```python
from build123d import *

# Parameters (mm, degrees)
F1_DEPTH       = 7
F3_DEPTH       = 5
F5_D           = 5.5
F5_CSINK_D     = 11.2
F5_CSINK_ANGLE = 90
F6_R           = 8
F7_R           = 3
F8_SIZE        = 1


with BuildPart() as f1:
    # F0 (on Top) → F1 (new body)
    with BuildSketch(Plane.XY):
        with BuildLine():
            Line((12.409673646, 7.5), (-12.409673646, 7.5))
            ThreePointArc((-12.409673646, 7.5), (-14.5, 0), (-12.409673646, -7.5))
            Line((-12.409673646, -7.5), (12.409673646, -7.5))
            ThreePointArc((12.409673646, -7.5), (14.5, 0), (12.409673646, 7.5))
        make_face()
    extrude(amount=F1_DEPTH)

    # F2 (on face) → F3 (join)
    with BuildSketch(Plane(origin=(0, 0, 0), x_dir=(1, 0, 0), z_dir=(0, 0, -1))):
        with BuildLine():
            Line((14.9666296342, 12.5000001863), (-14.9666296342, 12.5000001863))
            ThreePointArc((-14.9666296342, 12.5000001863), (-19.5000001863, 0), (-14.9666296342, -12.5000001863))
            Line((-14.9666296342, -12.5000001863), (14.9666296342, -12.5000001863))
            ThreePointArc((14.9666296342, -12.5000001863), (19.5000001863, 0), (14.9666296342, 12.5000001863))
        make_face()
        with BuildLine():
            Line((-12.409673646, 7.5), (12.409673646, 7.5))
            ThreePointArc((12.409673646, 7.5), (14.5, 0), (12.409673646, -7.5))
            Line((12.409673646, -7.5), (-12.409673646, -7.5))
            ThreePointArc((-12.409673646, -7.5), (-14.5, 0), (-12.409673646, 7.5))
        make_face(mode=Mode.SUBTRACT)
        with BuildLine():
            ThreePointArc((12.409673646, -7.5), (14.5, 0), (12.409673646, 7.5))
            Line((12.409673646, 7.5), (-12.409673646, 7.5))
            ThreePointArc((-12.409673646, 7.5), (-14.5, 0), (-12.409673646, -7.5))
            Line((-12.409673646, -7.5), (12.409673646, -7.5))
        make_face()
    extrude(amount=F3_DEPTH)

    # F5 (through all)
    with Locations(Plane(origin=(0, 0, -5), x_dir=(1, 0, 0), z_dir=(0, 0, -1))):
        with Locations((-8, 0), (8, 0)):
            CounterSinkHole(F5_D / 2, F5_CSINK_D / 2, counter_sink_angle=F5_CSINK_ANGLE)

    # F6
    f6_edges = [f1.edges().sort_by_distance(p)[0] for p in [
        (14.96663, -12.5, -2.5),
        (14.96663, 12.5, -2.5),
        (-14.96663, 12.5, -2.5),
        (-14.96663, -12.5, -2.5),
    ]]
    fillet(f6_edges, radius=F6_R)

    # F7
    f7_edges = [f1.edges().sort_by_distance(p)[0] for p in [
        (12.409674, -7.5, 3.5),
        (12.409674, 7.5, 3.5),
        (-12.409674, 7.5, 3.5),
        (-12.409674, -7.5, 3.5),
    ]]
    fillet(f7_edges, radius=F7_R)

    # F8
    f8_edges = [f1.edges().sort_by_distance(p)[0] for p in [
        (0, -12.5, -5),
        (-19.5, 0, -5),
        (0, 12.5, -5),
        (19.5, 0, -5),
        (19.5, 0, 0),
        (0, -12.5, 0),
        (-19.5, 0, 0),
        (0, 12.5, 0),
    ]]
    chamfer(f8_edges, length=F8_SIZE)


solid = f1.part
```
Design review of the part built by this model. Coordinates are the model's own, in mm. A direction names the side the tool comes from. Give positions to 0.01 mm unless a question says otherwise; leave off trailing zeros. Order: outer loops, then holes, each group sorted by start corner. A loop starts at its lowest first (then second) coordinate and runs counter-clockwise, first axis right, second up. Notation, with made-up numbers: M 21,-4 L 41,-4 A10 ccw 41,7 Z; hole C 5,-3 d4. An arc over 180 degrees is marked long. One line per question, with ' | ' between items. Start each with the question number.
Q1. For L1, parallel to Y at x = -8, z = 4; L2, parallel to Z at x = 5.5, y = 9; L3, parallel to Y at x = 9, z = 3, list the stretches that pass through material, from the lowest coordinate up. Write a range as [from, to].
Q2. We need section C-C (z = 3.75). Write out the cut boundary in (x, y), plus the area to 3 significant figures.
Q3. We need section D-D (z = -1.5). Write out the cut boundary in (x, y).
Q4. We need section A-A (y = 0). Write out the cut boundary in (x, z).
Q5. We need section B-B (x = 8). Write out the cut boundary in (y, z), plus the area to 3 significant figures.
Q6. For pin 1 Ø3 at (y, z) = (-1.5, 2) entering from +X; pin 2 Ø5.5 at (x, z) = (-0.5, 4) entering from -Y; pin 3 Ø3.5 at (x, z) = (3.5, 3.5) entering from +Y, all flat-tipped, find the tip position at first contact; note any pin that passes through.
Q7. The part is to be moulded in two halves that separate along Y. For faces 5 (the face through (-0.1, 12, -0.5)), 6 (the face through (0, 0, -5)), 7 (the face through (-10.54, 1.05, 2.49)), 8 (the face through (-19.5, -0.1, -2.5)), say which applies: +Y half, -Y half, draft (parallel to the pull), parting line (faces both ways), or undercut.
Q8. Machinability: for faces 1 (the face through (-14.5, 0.1, 3.5)), 2 (the face through (14.5, -0.1, 3.5)), 3 (the face through (12.258, 6.989, 3.549)), 4 (the face through (0, -7.5, 3)), which of the approach directions +Z, -Z, +X, -X, +Y, -Y give a long, thin tool a straight path to every point of the face, cutting with its end or side? Answer none if there is none.
Returned:
1) L1: [-7.5, -2.75], [2.75, 7.5] | L2: [-5, 0] | L3: [-7.5, -2.56], [2.56, 7.5]
2) outline: M -13.34,-5.67 A3 ccw -10.58,-7.5 L 10.58,-7.5 A3 ccw 13.34,-5.67 A14.5 ccw 13.34,5.67 A3 ccw 10.58,7.5 L -10.58,7.5 A3 ccw -13.34,5.67 A14.5 ccw Z; hole C -8,0 d5.5; hole C 8,0 d5.5 | area: 365 mm2
3) outline: M -17.95,-7.63 A8 ccw -10.58,-12.5 L 10.58,-12.5 A8 ccw 17.95,-7.63 A19.5 ccw 17.95,7.63 A8 ccw 10.58,12.5 L -10.58,12.5 A8 ccw -17.95,7.63 A19.5 ccw Z; hole C -8,0 d5.5; hole C 8,0 d5.5
4) outline: M -19.5,-4 L -18.5,-5 L -13.6,-5 L -10.75,-2.15 L -10.75,7 L -14.5,7 L -14.5,0 L -18.5,0 L -19.5,-1 Z; M -5.25,-2.15 L -2.4,-5 L 2.4,-5 L 5.25,-2.15 L 5.25,7 L -5.25,7 Z; M 10.75,-2.15 L 13.6,-5 L 18.5,-5 L 19.5,-4 L 19.5,-1 L 18.5,0 L 14.5,0 L 14.5,7 L 10.75,7 Z
5) outline: M -12.5,-4 L -11.5,-5 L -5.6,-5 L -2.75,-2.15 L -2.75,7 L -7.5,7 L -7.5,0 L -11.5,0 L -12.5,-1 Z; M 2.75,-2.15 L 5.6,-5 L 11.5,-5 L 12.5,-4 L 12.5,-1 L 11.5,0 L 7.5,0 L 7.5,7 L 2.75,7 Z | area: 154 mm2
6) pin 1: x = 14.5 | pin 2: y = -7.5 | pin 3: y = 7.5
7) face 5: +Y half | face 6: draft | face 7: undercut | face 8: parting line
8) face 1: +Z, -X | face 2: +Z, +X | face 3: +Z, +X, +Y | face 4: +Z, +X, -X, -Y
